Geometry: final body of the model. Coordinates: model frame, mm. A direction names the side the tool comes from. Give positions to 0.01 mm unless a question says otherwise; leave off trailing zeros. Order: outer loops, then holes, each group sorted by start corner. A loop starts at its lowest first (then second) coordinate and runs counter-clockwise, first axis right, second up. Notation, with made-up numbers: (14.25, -30) -> (52.25, -30) arc R20 cw to (52.25, -19) -> close; hole circle Ø1 at (78, 25.25). An arc over 180 degrees is marked (long way). One line per item, written item: value. Start each with the question number.
```python
from build123d import *

# Parameters (mm, degrees)
CHAMFER2_SIZE           = 0.5
SKETCH3_W               = 8
SKETCH3_H               = 2.4
CUT_EXTRUDE1_DEPTH      = 9.5
CUT_EXTRUDE1_DEPTH_BACK = 9.5


with BuildPart() as part:
    # Sketch2 → Revolve1 (revolve)
    with BuildSketch(Plane(origin=(0, 0, 0), x_dir=(1, 0, 0), z_dir=(0, 1, 0))):
        Polygon((0, 1.65), (-11, 1.65), (-11, 6.3), (-53, 6.3), (-53, 7.5), (-2, 7.5), (-2, 8.5), (0, 8.5), align=None)
    revolve(axis=Axis((0, 0, 0), (-1, 0, 0)))

    # Chamfer2
    chamfer2_edges = [part.edges().sort_by_distance(p)[0] for p in [
        (0, 0, 8.5),
        (0, 0, 1.65),
    ]]
    chamfer(chamfer2_edges, length=CHAMFER2_SIZE)

    # Sketch3 → Cut-Extrude1 (cut, two sides)
    with BuildSketch(Plane(origin=(0, 0, 0), x_dir=(1, 0, 0), z_dir=(0, 1, 0))) as cut_extrude1_sk:
        with Locations((-44, 0.817065344)):
            Rectangle(SKETCH3_W, SKETCH3_H)
    extrude(amount=CUT_EXTRUDE1_DEPTH, mode=Mode.SUBTRACT)
    extrude(cut_extrude1_sk.sketch, amount=-CUT_EXTRUDE1_DEPTH_BACK, mode=Mode.SUBTRACT)


solid = part.part
```
1. Pin query (flat end, axial travel): P1, Ø4, axis at y = 0, z = 0, coming from the +X side; P2, Ø3, axis at x = -37, z = -0.5, coming from the -Y side; P3, Ø1, axis at x = -43.5, y = -7, coming from the +Z side. Return the tip coordinate at first contact, or that it passes through.
2. Access query for faces 1 (the flat face through (-40, -7, -1)), 2 (the cylindrical face through (-27.143, -0.33, 7.493)), 3 (the flat face through (0, 2, -2)). Directions: +Z, -Z, +X, -X, +Y, -Y. A direction counts if a zero-diameter tool reaches every point of the face in a straight line with its end or side. Return the directions, or none.
3. Cut plane C-C, the plane x = -31.5. Return loops of the section in (y, z).
4. Cut plane B-B, the plane y = 0. Return loops of the section in (x, z).
5. Material intervals for L1, parallel to Y at x = -30, z = 0; L2, parallel to Y at x = -5.5, z = 0; L3, parallel to Z at x = -31, y = -0.5, sorted ascending. Write a range as [from, to].
6. Cut plane A-A, the plane x = -42. Return loops of the section in (y, z).
7. Draft query along Y for faces 4 (the cylindrical face through (-1.24, -7.167, -4.57)), 5 (the flat face through (-44, -7, 0.383)), 6 (the cylindrical face through (-32.29, 3.83, 5)). Return one class per face: pulls with the +Y half, pulls with the -Y half, needs draft (parallel to the pull), parting line crosses it, or undercut.
Answers follow:
1. P1: stops at x = -0.15
1. P2: stops at y = -7.5
1. P3: stops at z = 3.74
2. face 1: +Y, -Y
2. face 2: -X
2. face 3: +Z, -Z, +X, +Y, -Y
3. outline: circle Ø15 at (0, 0); hole circle Ø12.6 at (0, 0)
4. outline: (-53, -7.5) -> (-2, -7.5) -> (-2, -8.5) -> (-0.5, -8.5) -> (0, -8) -> (0, -2.15) -> (-0.5, -1.65) -> (-11, -1.65) -> (-11, -6.3) -> (-53, -6.3) -> close; (-53, 6.3) -> (-11, 6.3) -> (-11, 1.65) -> (-0.5, 1.65) -> (0, 2.15) -> (0, 8) -> (-0.5, 8.5) -> (-2, 8.5) -> (-2, 7.5) -> (-53, 7.5) -> close
5. L1: y = [-7.5, -6.3], [6.3, 7.5]
5. L2: y = [-7.5, -1.65], [1.65, 7.5]
5. L3: z = [-7.48, -6.28], [6.28, 7.48]
6. outline: (-7.49, 0.38) -> (-6.29, 0.38) arc R6.3 cw to (6.29, 0.38) -> (7.49, 0.38) arc R7.5 ccw to start; (-7.22, -2.02) arc R7.5 ccw to (7.22, -2.02) -> (5.97, -2.02) arc R6.3 cw to (-5.97, -2.02) -> close
7. face 4: parting line crosses it
7. face 5: needs draft
7. face 6: undercut
